from build123d import *

# Parameters (mm, degrees)
F3_D           = 6.6
F3_CSINK_D     = 13.44
F3_CSINK_ANGLE = 90


with BuildPart() as f1:
    # F0 (on Top) → F1 (revolve)
    with BuildSketch(Plane.XY):
        Polygon((-69, 5), (-69, -75), (-69, -80), (-61.5, -80), (0, -80), (0, -75), (-61.5, -75), (-61.5, 5), align=None)
    revolve(axis=Axis((0, -39.125, 0), (0, -1, 0)))

    # F3 (through all)
    with Locations(Plane(origin=(0, -75, 0), x_dir=(-1, 0, 0), z_dir=(0, 1, 0))):
        with Locations((14.45, 25.0281341694), (0, 0), (28.9, 0), (14.45, -25.0281341694), (-14.45, -25.0281341694), (-28.9, 0), (-14.45, 25.0281341694)):
            CounterSinkHole(F3_D / 2, F3_CSINK_D / 2, counter_sink_angle=F3_CSINK_ANGLE)


solid = f1.part
Read the model definition and answer for the solid it produces. Units are mm, in the model's axes. A direction names the side the tool comes from. Round coordinates to 2 decimals unless told otherwise and drop trailing zeros. Write each loop counter-clockwise with the first axis right and the second up, starting at its lowest first coordinate (ties: lowest second). Pieces come first, ordered by that corner, then holes.
1. The part is cut by section A-A, the plane z = 0. Determine the outline of the cut face in (x, y).
2. Determine the mould class of faces 3 (the face through (-65.814, -38.095, -20.726)), 4 (the face through (14.02, -79.221, -21.756)), 5 (the face through (-62, 5, 5)), 6 (the face through (14.02, -79.22, 28.3)) for opening direction Z: pulls with the +Z half, pulls with the -Z half, needs draft (parallel to the pull), parting line crosses it, or undercut.
3. The part is cut by section C-C, the plane x = -14.45. Determine the outline of the cut face in (y, z), then the cut area to 3 significant figures.
4. The part is cut by section D-D, the plane y = -20.5. Determine the outline of the cut face in (x, z).
5. Straight lines are drawn through the part: L1, parallel to Z at x = 0, y = -53; L2, parallel to Z at x = 14.45, y = -79.45. For each, find the intervals that lie inside material, in ascending order.
6. Given pin 1 Ø1.5 at (x, y) = (-8, -53.5) entering from +Z; pin 2 Ø3 at (y, z) = (-40, 9) entering from +X; pin 3 Ø6 at (x, z) = (-14.45, -25.03) entering from +Y; pin 4 Ø12 at (x, y) = (-54, -53.5) entering from -Z, each flat-ended and moving along its own axis, determine where each tip first touches the part or whether it passes through.
7. The part is cut by section B-B, the plane x = 0. Determine the outline of the cut face in (y, z), then the cut area to 3 significant figures.
8. Which of the six approach directions +Z, -Z, +X, -X, +Y, -Y give full straight-line access (tool end or side, diameter ignored) to faces 1 (the face through (32.05, -79.22, 0.99)), 2 (the face through (13, -75, -1))?
Values:
1. outline: (-69, -80) - (-32.2, -80) - (-32.2, -78.42) - (-35.62, -75) - (-61.5, -75) - (-61.5, 5) - (-69, 5) - close; (-25.6, -80) - (-3.3, -80) - (-3.3, -78.42) - (-6.72, -75) - (-22.18, -75) - (-25.6, -78.42) - close; (3.3, -80) - (25.6, -80) - (25.6, -78.42) - (22.18, -75) - (6.72, -75) - (3.3, -78.42) - close; (32.2, -80) - (69, -80) - (69, 5) - (61.5, 5) - (61.5, -75) - (35.62, -75) - (32.2, -78.42) - close
2. face 3: parting line crosses it
2. face 4: undercut
2. face 5: needs draft
2. face 6: undercut
3. outline: (-80, -67.47) - (5, -67.47) - (5, -59.78) - (-75, -59.78) - (-75, -31.75) - (-78.42, -28.33) - (-80, -28.33) - close; (-80, -21.73) - (-78.42, -21.73) - (-75, -18.31) - (-75, 18.31) - (-78.42, 21.73) - (-80, 21.73) - close; (-80, 28.33) - (-78.42, 28.33) - (-75, 31.75) - (-75, 59.78) - (5, 59.78) - (5, 67.47) - (-80, 67.47) - close
3. area: 1,820 mm2
4. outline: circle Ø138 at (0, 0); hole circle Ø123 at (0, 0)
5. L1: z = -69 to -61.5, 61.5 to 69
5. L2: z = -67.47 to -28.33, -21.73 to 21.73, 28.33 to 67.47
6. pin 1: stops at z = 68.62
6. pin 2: stops at x = 68.59
6. pin 3: passes through
6. pin 4: stops at z = -49.57
7. outline: (-80, -69) - (5, -69) - (5, -61.5) - (-75, -61.5) - (-75, -6.72) - (-78.42, -3.3) - (-80, -3.3) - close; (-80, 3.3) - (-78.42, 3.3) - (-75, 6.72) - (-75, 61.5) - (5, 61.5) - (5, 69) - (-80, 69) - close
7. area: 1,850 mm2
8. face 1: +Y, -Y
8. face 2: +Y
